```python
from build123d import *

# Parameters (mm, degrees)
BOSS_EXTRUDE1_DEPTH     = 10
SKETCH2_W               = 16
SKETCH2_H               = 14
CUT_EXTRUDE1_DEPTH      = 10
BOSS_EXTRUDE2_DEPTH     = 2.5
CUT_EXTRUDE_THIN1_START = -32.5
SKETCH3_4_R             = 40
SKETCH3_4_R_2           = 30
CUT_EXTRUDE_THIN1_DEPTH = 32.5


with BuildPart() as part:
    # Sketch1 → Boss-Extrude1 (new, symmetric)
    with BuildSketch(Plane(origin=(0, 0, 0), x_dir=(1, 0, 0), z_dir=(0, 1, 0))):
        Polygon((15, 10), (-15, 10), (-15, -10), align=None)
    extrude(amount=BOSS_EXTRUDE1_DEPTH, both=True)

    # Sketch2 → Cut-Extrude1 (cut, symmetric)
    with BuildSketch(Plane(origin=(0, 0, 0), x_dir=(0, 0, -1), z_dir=(1, 0, 0))):
        Rectangle(SKETCH2_W, SKETCH2_H)
    extrude(amount=CUT_EXTRUDE1_DEPTH, both=True, mode=Mode.SUBTRACT)

    # Sketch3 → Boss-Extrude2 (add)
    with BuildSketch(Plane.ZY.offset(15)):
        with BuildLine():
            ThreePointArc((8.284271247, 10), (3.070072037, 19.177376677), (-5, 25.980762114))
            Line((-5, 25.980762114), (-5, 10))
            Line((-5, 10), (8.284271247, 10))
        make_face()
        with BuildLine():
            Line((8.284271247, -10), (-5, -10))
            Line((-5, -10), (-5, -25.980762114))
            ThreePointArc((-5, -25.980762114), (3.070072037, -19.177376677), (8.284271247, -10))
        make_face()
        with BuildLine():
            Line((8.284271247, 10), (-5, 10))
            Line((-5, 10), (-5, -10))
            Line((-5, -10), (8.284271247, -10))
            ThreePointArc((8.284271247, -10), (9.56795679, -5.073059362), (10, 0))
            ThreePointArc((10, 0), (9.56795679, 5.073059362), (8.284271247, 10))
        make_face()
    extrude(amount=BOSS_EXTRUDE2_DEPTH)

    # Sketch3_4 → Cut-Extrude-Thin1 (cut)
    with BuildSketch(Plane.ZY.offset(15).offset(CUT_EXTRUDE_THIN1_START)):
        with Locations((-20, 0)):
            Circle(SKETCH3_4_R)
        with Locations((-20, 0)):
            Circle(SKETCH3_4_R_2, mode=Mode.SUBTRACT)
    extrude(amount=CUT_EXTRUDE_THIN1_DEPTH, mode=Mode.SUBTRACT)


solid = part.part
```
Here's how the part is built. I have some questions about the finished solid (model axes, mm). A direction names the side the tool comes from. Give positions to 0.01 mm unless a question says otherwise; leave off trailing zeros. Write each loop counter-clockwise with the first axis right and the second up, starting at its lowest first coordinate (ties: lowest second). Pieces come first, ordered by that corner, then holes.
(1) Imagine slicing it at A-A, the plane z = -6. Write out the boundary of the cut face in (x, y), and give its area (3 significant figures).
Output values:
outline: (-15, -10) - (9, -10) - (9, -7) - (-10, -7) - (-10, 7) - (9, 7) - (9, 10) - (-15, 10) - close
area: 214 mm2
(2) Imagine slicing it at D-D, the plane z = 5.5. Write out the boundary of the cut face in (x, y), and give its area (3 significant figures).
Output values:
outline: (-17.5, -15.8) - (-15, -15.8) - (-15, -10) - (-8.25, -10) - (-8.25, -7) - (-10, -7) - (-10, 7) - (-8.25, 7) - (-8.25, 10) - (-15, 10) - (-15, 15.8) - (-17.5, 15.8) - close
area: 190 mm2
(3) Imagine slicing it at C-C, the plane x = 4. Write out the boundary of the cut face in (y, z), and give its area (3 significant figures).
Output values:
outline: (-10, -10) - (10, -10) - (10, -2.67) - (7, -2.67) - (7, -8) - (-7, -8) - (-7, -2.67) - (-10, -2.67) - close
area: 72.0 mm2
(4) On a 3-axis mill with a long thin cutter (end or side, diameter ignored), from which of +Z, -Z, +X, -X, +Y, -Y can I reach the whole of each face in a straight line? I mean faces 1 (the face through (-16, 0, -5)), 2 (the face through (-4, -10, -3)), 3 (the face through (10, 0, -7)), 4 (the face through (-4, 10, -3)). Say none if no direction works.
Output values:
face 1: -Z, -X, +Y, -Y
face 2: +Z, -Z, +X, -Y
face 3: +Z
face 4: +Z, -Z, +X, +Y
(5) Will these pins go through, and if not, where does the flat tip stop? pin 1 (4 mm diameter, centred on x = -7.5, z = -4, fed in from +Y); pin 2 (2.5 mm diameter, centred on y = 3, z = -7.5, fed in from -X); pin 3 (4.5 mm diameter, centred on x = -2, z = -1.5, fed in from -Y).
Output values:
pin 1: stops at y = 10
pin 2: stops at x = -15
pin 3: stops at y = -10
(6) Imagine slicing it at B-B, the plane y = 8.5. Write out the boundary of the cut face in (x, z).
Output values:
outline: (-17.5, -5) - (-15, -5) - (-15, -10) - (15, -10) - (-13.16, 8.77) - (-17.5, 8.77) - close
(7) If I drill on L1, parallel to Y at x = -9.5, z = -1.75; L2, parallel to Z at x = -10, y = -9; L3, parallel to X at y = -19, z = 1.5, over which ranges is the centre line in solid material (lowest first)?
Output values:
L1: y = -10 to -7, 7 to 10
L2: z = -10 to 6.67
L3: x = -17.5 to -15
(8) Thinking about a two-plate mould opening in X: for faces 5 (the face through (-15, 16, 0)), 6 (the face through (0, 0, -8)), 7 (the face through (0, 0, -10)), which applies, pulls with the +X half, pulls with the -X half, needs draft (parallel to the pull), parting line crosses it, or undercut?
Output values:
face 5: pulls with the +X half
face 6: undercut
face 7: needs draft
